The model under review builds one solid part; all positions refer to its coordinate system, in mm. A direction names the side the tool comes from. Round coordinates to 2 decimals unless told otherwise and drop trailing zeros. Loops run counter-clockwise (first coordinate to the right, second up) from the corner with the lowest first, then second, coordinate; pieces in that order, holes last. Notation, with made-up numbers: M 54,50 L 67,50 A15 ccw 67,57 Z; hole C 63.5,82 d2. An arc over 180 degrees is marked long. Answer in a Markdown table with one row per item. Add a question column.
from build123d import *

# Parameters (mm, degrees)
BOSS_EXTRUDE1_DEPTH = 63
CUT_EXTRUDE1_DEPTH  = 15
BOSS_EXTRUDE2_DEPTH = 25
CUT_EXTRUDE2_DEPTH  = 19


with BuildPart() as part:
    # Sketch1 → Boss-Extrude1 (new body)
    with BuildSketch(Plane(origin=(0, 0, 0), x_dir=(0, 0, -1), z_dir=(1, 0, 0))):
        Polygon((75, 0), (75, 50), (0, 12), (0, 0), align=None)
    extrude(amount=-BOSS_EXTRUDE1_DEPTH)

    # Sketch2 → Cut-Extrude1 (cut)
    with BuildSketch(Plane(origin=(0, 0, 0), x_dir=(0, 0, -1), z_dir=(1, 0, 0))):
        Polygon((50, 0), (50, 37.333333333), (25, 24.666666667), (25, 0), align=None)
    extrude(amount=-CUT_EXTRUDE1_DEPTH, mode=Mode.SUBTRACT)

    # Sketch4 → Boss-Extrude2 (add)
    with BuildSketch(Plane(origin=(-19, 0, 0), x_dir=(0, 0, -1), z_dir=(1, 0, 0))):
        Polygon((12, 18.08), (12, 34.08), (43.578947368, 34.08), align=None)
    extrude(amount=-BOSS_EXTRUDE2_DEPTH)

    # Sketch5 → Cut-Extrude2 (cut)
    with BuildSketch(Plane(origin=(-22, 0, 0), x_dir=(0, 0, -1), z_dir=(1, 0, 0))):
        Polygon((75, 50), (50, 37.333333333), (75, 37.333333333), align=None)
    extrude(amount=-CUT_EXTRUDE2_DEPTH, mode=Mode.SUBTRACT)


solid = part.part
1. Mouldability with a two-part tool opening along Z and no side actions: class faces 4 (the flat face through (-44, 30, -21)), 5 (the flat face through (-7, 18, -50)), 6 (the flat face through (-31, 6, 0)), 7 (the flat face through (-15, 15, -37)) as released by +Z, released by -Z, zero draft, split by the parting line, or undercut.
2. Take a section at A-A, the plane z = -42. State the section outline as (x, y) points.
3. Take a section at C-C, the plane y = 42.5. State the section outline as (x, z) points.
4. Take a section at B-B, the plane x = -6. State the section outline as (y, z) points.
5. To check wall thickness, follow probe 1 along Z at (x, y) = (-3.5, 7.5); probe 2 along Z at (x, y) = (-9, 28.5); probe 3 along Y at (x, z) = (-22, -18). State the ranges of each line that lie inside material, in increasing order.
6. Machinability: for faces 1 (the flat face through (-41, 41, -68)), 2 (the flat face through (-31, 34.08, -28)), 3 (the flat face through (-19, 30, -21)), which of the approach directions +Z, -Z, +X, -X, +Y, -Y give a long, thin tool a straight path to every point of the face, cutting with its end or side? Answer none if there is none.
7. Take a section at D-D, the plane x = -25. State the section outline as (y, z) points.
8. For pin 1 Ø9.5 at (x, z) = (-30.5, -63.5) entering from +Y; pin 2 Ø4 at (x, y) = (-40.5, 31) entering from +Z; pin 3 Ø10 at (x, z) = (-25.5, -53) entering from +Y, all flat-tipped, find the tip position at first contact; note any pin that passes through.
Check sheet entries:
| question | item | result |
|---|---|---|
| 1 | face 4 | zero draft |
| 1 | face 5 | undercut |
| 1 | face 6 | released by +Z |
| 1 | face 7 | undercut |
| 2 | outline | M -63,0 L -15,0 L -15,33.28 L -19,33.28 L -19,34.08 L -44,34.08 L -44,33.28 L -63,33.28 Z |
| 3 | outline | M -63,-75 L -41,-75 L -41,-60.2 L -63,-60.2 Z; M -22,-75 L 0,-75 L 0,-60.2 L -22,-60.2 Z |
| 4 | outline | M 0,-75 L 50,-75 L 37.33,-50 L 0,-50 Z; M 0,-25 L 24.67,-25 L 12,0 L 0,0 Z |
| 5 | probe 1 | z = -75 to -50, -25 to 0 |
| 5 | probe 2 | z = -75 to -50 |
| 5 | probe 3 | y = 0 to 34.08 |
| 6 | face 1 | +Z, -Z, +Y |
| 6 | face 2 | +Z, +X, -X, +Y |
| 6 | face 3 | +Z, +X, +Y |
| 7 | outline | M 0,-75 L 37.33,-75 L 37.33,-50 L 34.08,-43.58 L 34.08,-12 L 18.08,-12 L 12,0 L 0,0 Z |
| 8 | pin 1 | stops at y = 37.33 |
| 8 | pin 2 | stops at z = -12 |
| 8 | pin 3 | stops at y = 40.66 |
